Here's how the part is built. I have some questions about the finished solid (model axes, mm). Face numbers are marked on the shaded views. Give positions to 0.01 mm unless a question says otherwise; leave off trailing zeros. Loops run counter-clockwise (first coordinate to the right, second up) from the corner with the lowest first, then second, coordinate; pieces in that order, holes last. Notation, with made-up numbers: (5, 75) -> (31, 75) arc R21 ccw to (31, 103) -> close; hole circle Ø9 at (82, -2.75). An arc over 180 degrees is marked (long way). Answer in a Markdown table with one row per item. Add a question column.
Item 1: If I drill on line 1 (Y direction, x = 0, z = 22); line 2 (Z direction, x = 52, y = 0); line 3 (X direction, y = 0, z = 17.5), over which ranges is the centre line in solid material (lowest first)?
Item 2: If we section it at A-A (y = 0): Write out the boundary of the cut face in (x, z).
Item 3: We'd pull the mould along X, two halves only. Please class the marked faces 1, 2 and 3: released by +X, released by -X, zero draft, split by the parting line, or undercut.
Item 4: If we section it at B-B (x = 87.5): Write out the boundary of the cut face in (y, z), then the cut area to 3 significant figures.
Item 5: If we section it at C-C (z = 15): Write out the boundary of the cut face in (x, y), then the cut area to 3 significant figures.
Item 6: If we section it at D-D (x = 20.5): Write out the boundary of the cut face in (y, z).
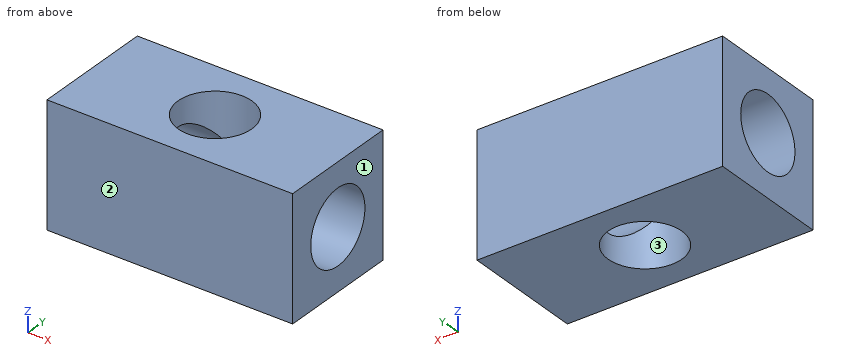
```python
from build123d import *

# Parameters (mm, degrees)
F0_W     = 200
F0_H     = 100
F1_DEPTH = 100
F2_R     = 30
F3_DEPTH = 100
F4_R     = 30
F5_DEPTH = 200.001


with BuildPart() as f1:
    # F0 (on Top) → F1 (new body)
    with BuildSketch(Plane.XY):
        Rectangle(F0_W, F0_H)
    extrude(amount=F1_DEPTH)

    # F2 (on face) → F3 (cut, through all)
    with BuildSketch(Plane.XY.offset(100)):
        Circle(F2_R)
    extrude(amount=-F3_DEPTH, mode=Mode.SUBTRACT)

    # F4 (on face) → F5 (cut, through all)
    with BuildSketch(Plane.YZ.offset(100)):
        with Locations((0, 50)):
            Circle(F4_R)
    extrude(amount=-F5_DEPTH, mode=Mode.SUBTRACT)


solid = f1.part
```
Recorded:
| question | item | result |
|---|---|---|
| 1 | line 1 | y = -50 to -30, 30 to 50 |
| 1 | line 2 | z = 0 to 20, 80 to 100 |
| 1 | line 3 | x = -100 to -30, 30 to 100 |
| 2 | outline | (-100, 0) -> (-30, 0) -> (-30, 20) -> (-100, 20) -> close; (-100, 80) -> (-30, 80) -> (-30, 100) -> (-100, 100) -> close; (30, 0) -> (100, 0) -> (100, 20) -> (30, 20) -> close; (30, 80) -> (100, 80) -> (100, 100) -> (30, 100) -> close |
| 3 | face 1 | released by +X |
| 3 | face 2 | zero draft |
| 3 | face 3 | undercut |
| 4 | outline | (-50, 0) -> (50, 0) -> (50, 100) -> (-50, 100) -> close; hole circle Ø60 at (0, 50) |
| 4 | area | 7,170 mm^2 |
| 5 | outline | (-100, -50) -> (100, -50) -> (100, 50) -> (-100, 50) -> close; hole circle Ø60 at (0, 0) |
| 5 | area | 17,200 mm^2 |
| 6 | outline | (-50, 0) -> (-21.9, 0) -> (-21.9, 29.5) arc R30 cw to (-21.9, 70.5) -> (-21.9, 100) -> (-50, 100) -> close; (21.9, 0) -> (50, 0) -> (50, 100) -> (21.9, 100) -> (21.9, 70.5) arc R30 cw to (21.9, 29.5) -> close |
